Verification items for the finished model (mm, model axes). Face numbers are marked on the shaded views. A direction names the side the tool comes from. Give positions to 0.01 mm unless a question says otherwise; leave off trailing zeros. Write each loop counter-clockwise with the first axis right and the second up, starting at its lowest first coordinate (ties: lowest second). Pieces come first, ordered by that corner, then holes. Notation, with made-up numbers: M -11.75,48.25 L 32.25,48.25 A29 ccw 32.25,75.25 Z; hole C -13.5,49 d10. An arc over 180 degrees is marked long. Write item = value, one per line.
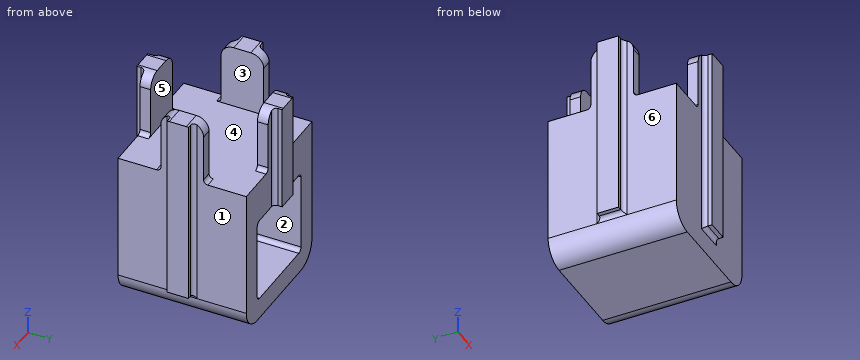
from build123d import *

# Parameters (mm, degrees)
SKETCH1_W           = 30
SKETCH1_H           = 30
BOSS_EXTRUDE1_DEPTH = 35
SKETCH2_W           = 20
SKETCH2_H           = 20
CUT_EXTRUDE1_DEPTH  = 20
SKETCH3_W           = 10
SKETCH3_H           = 2.5
SKETCH3_W_2         = 2.5
SKETCH3_H_2         = 10
BOSS_EXTRUDE2_DEPTH = 15
FILLET3_R           = 5
SKETCH4_W           = 44
SKETCH4_H           = 5
BOSS_EXTRUDE3_DEPTH = 2
CIRPATTERN1_COUNT   = 3
CIRPATTERN1_ANGLE   = 180
SKETCH5_W           = 5
SKETCH5_H           = 25
BOSS_EXTRUDE4_DEPTH = 2
FILLET1_R           = 1
FILLET2_R           = 3


with BuildPart() as part:
    # Sketch1 → Boss-Extrude1 (new body)
    with BuildSketch(Plane.XY):
        Rectangle(SKETCH1_W, SKETCH1_H)
    extrude(amount=BOSS_EXTRUDE1_DEPTH)

    # Sketch2 → Cut-Extrude1 (cut)
    with BuildSketch(Plane(origin=(0, 15, 0), x_dir=(1, 0, 0), z_dir=(0, 1, 0))):
        with Locations((0, -15)):
            Rectangle(SKETCH2_W, SKETCH2_H)
    extrude(amount=-CUT_EXTRUDE1_DEPTH, mode=Mode.SUBTRACT)

    # Sketch3 → Boss-Extrude2 (add)
    with BuildSketch(Plane.XY.offset(35)):
        with Locations((0, 13.75)):
            Rectangle(SKETCH3_W, SKETCH3_H)
        with Locations((13.75, 0)):
            Rectangle(SKETCH3_W_2, SKETCH3_H_2)
        with Locations((0, -13.75)):
            Rectangle(SKETCH3_W, SKETCH3_H)
        with Locations((-13.75, 0)):
            Rectangle(SKETCH3_W_2, SKETCH3_H_2)
    extrude(amount=BOSS_EXTRUDE2_DEPTH)

    # Fillet3
    fillet3_edges = [part.edges().sort_by_distance(p)[0] for p in [
        (15, 0, 0),
        (-15, 0, 0),
    ]]
    fillet(fillet3_edges, radius=FILLET3_R)

    # Sketch4 → Boss-Extrude3 (add)
    with BuildSketch(Plane(origin=(15, 0, 0), x_dir=(0, 0, -1), z_dir=(1, 0, 0))):
        with Locations((-28, 0)):
            Rectangle(SKETCH4_W, SKETCH4_H)
    boss_extrude3 = extrude(amount=BOSS_EXTRUDE3_DEPTH)

    # CirPattern1: Boss-Extrude3 ×3 about axis
    cirpattern1_axis = Axis((0, 0, 0), (0, 0, -1))
    for i in range(1, CIRPATTERN1_COUNT):
        add(boss_extrude3.rotate(cirpattern1_axis, i * CIRPATTERN1_ANGLE / (CIRPATTERN1_COUNT - 1)))

    # Sketch5 → Boss-Extrude4 (add)
    with BuildSketch(Plane(origin=(0, 15, 0), x_dir=(1, 0, 0), z_dir=(0, 1, 0))):
        with Locations((0, -37.5)):
            Rectangle(SKETCH5_W, SKETCH5_H)
    extrude(amount=BOSS_EXTRUDE4_DEPTH)

    # Fillet1
    fillet1_edges = [part.edges().sort_by_distance(p)[0] for p in [
        (-2.5, -15, 28),
        (0, -15, 6),
        (2.5, -15, 28),
        (-15, 2.5, 28),
        (-15, 0, 6),
        (-15, -2.5, 28),
        (-2.5, 15, 37.5),
        (2.5, 15, 37.5),
        (-10, 5, 25),
        (-10, 5, 5),
        (10, 5, 5),
        (10, 5, 25),
        (-5, 13.75, 35),
        (5, 13.75, 35),
        (13.75, 5, 35),
        (13.75, -5, 35),
        (5, -13.75, 35),
        (-5, -13.75, 35),
        (-13.75, -5, 35),
        (-13.75, 5, 35),
        (15, -2.5, 28),
        (15, 0, 6),
        (15, 2.5, 28),
    ]]
    fillet(fillet1_edges, radius=FILLET1_R - 0.0001)  # a hair under: the kernel refuses the full size

    # Fillet2
    fillet2_edges = [part.edges().sort_by_distance(p)[0] for p in [
        (-13.75, 5, 50),
        (-13.75, -5, 50),
        (5, -13.75, 50),
        (-5, -13.75, 50),
        (13.75, -5, 50),
        (13.75, 5, 50),
        (5, 13.75, 50),
        (-5, 13.75, 50),
    ]]
    fillet(fillet2_edges, radius=FILLET2_R)


solid = part.part
1) Draft check along X on the marked faces 4, 5 and 6. Enter one of: +X half, -X half, draft (parallel to the pull), parting line (faces both ways), or undercut.
From the geometry:
face_4 = undercut
face_5 = draft
face_6 = -X half
2) Cross-section at A-A on y = 13.5. Record the boundary of the cut face in (x, z), plus the area to 3 significant figures.
From the geometry:
outline = M -15,5 A5 ccw -10,0 L 10,0 A5 ccw 15,5 L 15,35 L 6,35 A1 cw 5,36 L 5,47 A3 ccw 2,50 L -2,50 A3 ccw -5,47 L -5,36 A1 cw -6,35 L -15,35 Z; hole M -10,6 A1 ccw -9,5 L 9,5 A1 ccw 10,6 L 10,24 A1 ccw 9,25 L -9,25 A1 ccw -10,24 Z
area = 787 mm^2
3) Cross-section at C-C on x = -14. Record the boundary of the cut face in (y, z), plus the area to 3 significant figures.
From the geometry:
outline = M -15,2 L 15,2 L 15,35 L 6,35 A1 cw 5,36 L 5,47 A3 ccw 2,50 L -2,50 A3 ccw -5,47 L -5,36 A1 cw -6,35 L -15,35 Z
area = 1,140 mm^2
4) Cross-section at B-B on z = 44.5. Count the separate pieces of the cut face and the enclosed holes in it, plus the area to 3 significant figures.
From the geometry:
separate_pieces = 4
enclosed_holes = 0
area = 142 mm^2
5) Depth check by flat-ended pin: P1, Ø1.1, axis at x = 16.5, y = 0, coming from the -Z side; P2, Ø1, axis at x = 12.5, y = -8, coming from the +Z side; P3, Ø4, axis at x = 5.5, z = 42, coming from the +Y side. Enter the tip coordinate at first touch or a pass-through.
From the geometry:
P1 = 6
P2 = 35
P3 = 15
6) Cross-section at D-D on z = 32.5. Record the boundary of the cut face in (x, y), plus the area to 3 significant figures.
From the geometry:
outline = M -17,-2.5 L -16,-2.5 A1 cw -15,-3.5 L -15,-15 L -3.5,-15 A1 cw -2.5,-16 L -2.5,-17 L 2.5,-17 L 2.5,-16 A1 cw 3.5,-15 L 15,-15 L 15,-3.5 A1 cw 16,-2.5 L 17,-2.5 L 17,2.5 L 16,2.5 A1 cw 15,3.5 L 15,15 L 3.5,15 A1 cw 2.5,16 L 2.5,17 L -2.5,17 L -2.5,16 A1 cw -3.5,15 L -15,15 L -15,3.5 A1 cw -16,2.5 L -17,2.5 Z
area = 942 mm^2
7) Material ranges on probe 1 along X at (y, z) = (14.5, 18); probe 2 along Z at (x, y) = (9, -3.5); probe 3 along X at (y, z) = (0.5, 11), recorded low to high. Write a range as from..to.
From the geometry:
probe_1 = -15..-10, 10..15
probe_2 = 0..5, 25..35
probe_3 = -17..-10, 10..17
8) Tool access check on the marked faces 1, 2 and 3. Record the directions out of +Z, -Z, +X, -X, +Y, -Y that give a thin tool (end or side, any length) a straight path to the whole face; none if there is none.
From the geometry:
face_1 = +Z, -Z, +X
face_2 = +Y
face_3 = +Z, +Y, -Y
